Input: dimensioned drawing with shaded views. Units: mm. Origin: part minimum x, y, z. A direction names the side the tool comes from. Give positions to 0.01 mm unless a question says otherwise; leave off trailing zeros. Write each loop counter-clockwise with the first axis right and the second up, starting at its lowest first coordinate (ties: lowest second). Pieces come first, ordered by that corner, then holes. Notation, with made-up numbers: (63.25, 67) -> (68.25, 67) arc R22 cw to (68.25, 99) -> close; hole circle Ø2 at (29.5, 72). An arc over 180 degrees is marked (long way). Answer as a JSON object with one key per item and string values.
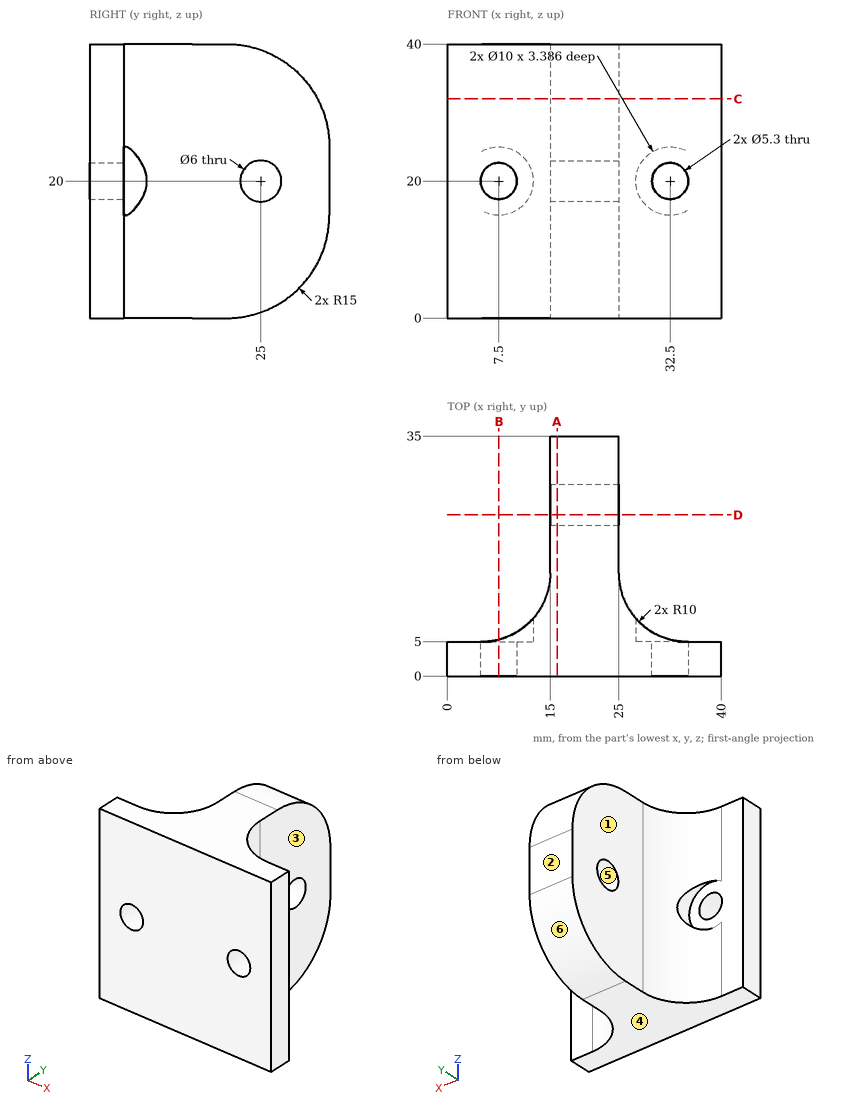
Q1. Mould query, pull axis Y, two halves, no side actions, for the marked faces 4, 5 and 6. Classes: pulls with the +Y half, pulls with the -Y half, needs draft (parallel to the pull), parting line crosses it, or undercut.
Values:
{"face 4": "needs draft", "face 5": "undercut", "face 6": "pulls with the +Y half"}
Q2. First-contact query: P1, Ø11.5, axis at x = 32.5, z = 20, coming from the +Y side; P2, Ø6, axis at x = 4.5, z = 5.5, coming from the +Y side; P3, Ø10, axis at x = 5.5, z = 15.5, coming from the +Y side. Flat tips, straight axial feed; report the tip coordinate or a pass-through.
Values:
{"P1": "y = 9.35", "P2": "y = 5.32", "P3": "y = 6.65"}
Q3. Cut plane D-D (y = 23.5). Return the cut outline in (x, z).
Values:
{"outline": "(15, 0.41) -> (25, 0.41) -> (25, 17.4) -> (15, 17.4) -> close; (15, 22.6) -> (25, 22.6) -> (25, 39.59) -> (15, 39.59) -> close"}
Q4. Material intervals for L1, parallel to X at y = 16.5, z = 30; L2, parallel to Z at x = 7, y = 3; L3, parallel to Y at x = 3, z = 30, sorted ascending. Write a range as from..to.
Values:
{"L1": "15..25", "L2": "0..17.4, 22.6..40", "L3": "0..5"}
Q5. Cut plane C-C (z = 32). Return the cut outline in (x, y).
Values:
{"outline": "(0, 0) -> (40, 0) -> (40, 5) -> (35, 5) arc R10 cw to (25, 15) -> (25, 33.27) -> (15, 33.27) -> (15, 15) arc R10 cw to (5, 5) -> (0, 5) -> close"}
Q6. Cut plane B-B (x = 7.5). Return the cut outline in (y, z), and give its area (3 significant figures).
Values:
{"outline": "(0, 0) -> (5.32, 0) -> (5.32, 15) -> (5, 15) -> (5, 17.35) -> (0, 17.35) -> close; (0, 22.65) -> (5, 22.65) -> (5, 25) -> (5.32, 25) -> (5.32, 40) -> (0, 40) -> close", "area": "183 mm²"}
Q7. Cut plane A-A (x = 16). Return the cut outline in (y, z).
Values:
{"outline": "(0, 0) -> (20, 0) arc R15 ccw to (35, 15) -> (35, 25) arc R15 ccw to (20, 40) -> (0, 40) -> close; hole circle Ø6 at (25, 20)"}
Q8. Set-up query: the marked faces 1, 2 and 3. Return all of +Z, -Z, +X, -X, +Y, -Y with unobstructed straight access to the full face (end or side cutting, diameter ignored); none if empty.
Values:
{"face 1": "+Z, -Z, -X, +Y", "face 2": "+Z, -Z, +X, -X, +Y", "face 3": "+Z, -Z, +X, +Y"}
